Here's the drawing with two shaded views (mm, measured from the low corner). I have some questions. A direction names the side the tool comes from. Coordinates: 2 decimals unless noted, no trailing zeros. Write each loop counter-clockwise with the first axis right and the second up, starting at its lowest first coordinate (ties: lowest second). Pieces come first, ordered by that corner, then holes. Notation, with made-up numbers: (-14.75, 9) -> (-2.75, 9) arc R26 cw to (-2.75, 27) -> close; hole circle Ø5 at (22.5, 80). An arc over 180 degrees is marked (long way). Put each result on its own line as item: value. Start each with the question number.
Item 1: I want a section at C-C, the plane z = 35.5. List the corners of the cut face in (x, y) for me, then the cut area to 3 significant figures.
Item 2: If we mould it in two halves opening along Y, with no side actions, what happens to the marked faces 3, 4 and 5? For each: released by +Y, released by -Y, zero draft, split by the parting line, or undercut.
Item 3: I need wall thicknesses on line 1 (Z direction, x = 14.25, y = 75); line 2 (Z direction, x = 4.5, y = 100); line 3 (Y direction, x = 17.75, z = 50). Which ranges of each line are inside material? Lowest first, please. Write a range as [from, to].
Item 4: On a 3-axis mill with a long thin cutter (end or side, diameter ignored), from which of +Z, -Z, +X, -X, +Y, -Y can I reach the whole of each face in a straight line? I mean the marked faces 1 and 2. Say none if no direction works.
Item 5: I want a section at B-B, the plane x = 11.5. State how many separate pieces and enclosed holes the cut face has, then the cut area to 3 significant figures.
Item 6: I want a section at A-A, the plane x = 17.75. List the corners of the cut face in (y, z) for me.
Item 7: For pin 1 (9.5 mm diameter, centred on y = 50, z = 75, fed in from +X); pin 2 (11 mm diameter, centred on y = 100, z = 100, fed in from -X); pin 3 (4 mm diameter, centred on x = 17.5, z = 60, fed in from +Y), each with a flat end and sliding along its axis, tell me the tip position at first contact or that it passes through.
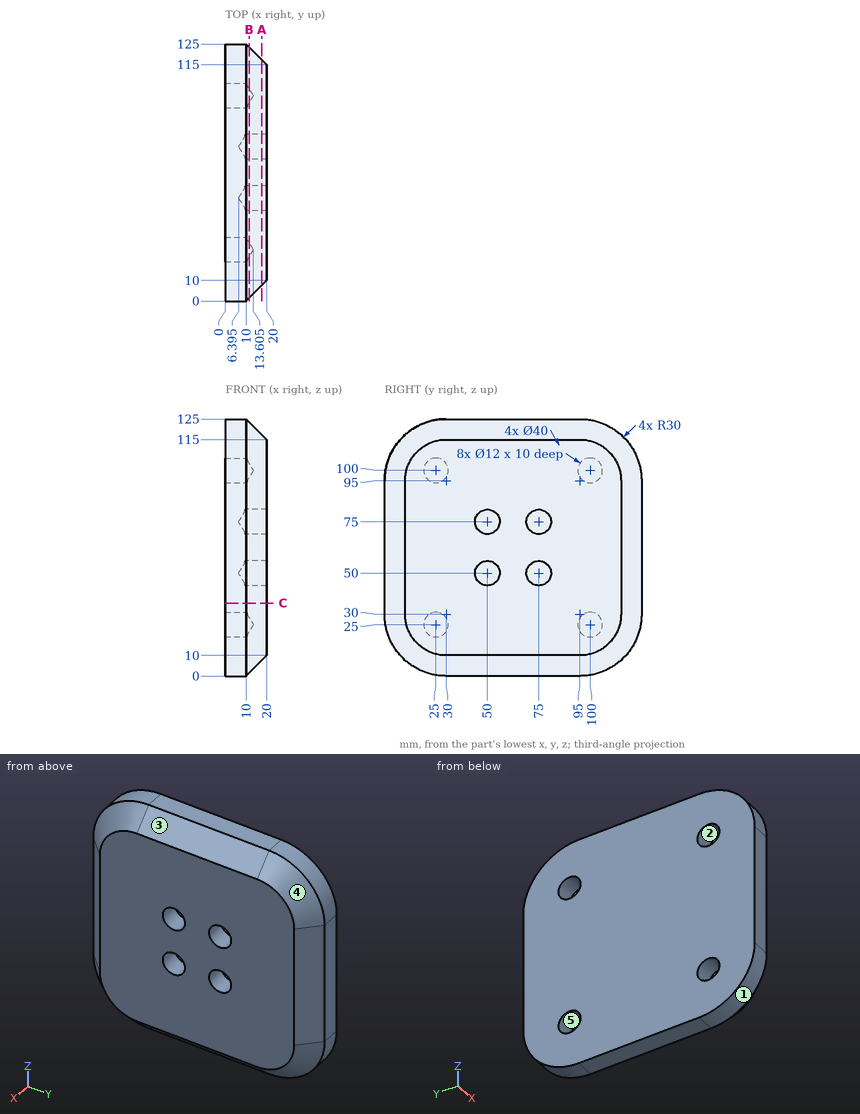
Calculated:
1. outline: (0, 0) -> (10, 0) -> (20, 10) -> (20, 115) -> (10, 125) -> (0, 125) -> close
1. area: 2,400 mm2
2. face 3: zero draft
2. face 4: released by +Y
2. face 5: undercut
3. line 1: z = [4.25, 44], [56, 69], [81, 120.75]
3. line 2: z = [0.42, 19], [31, 94], [106, 124.58]
3. line 3: y = [7.75, 44], [56, 69], [81, 117.25]
4. face 1: -Z, +X, -X, -Y
4. face 2: -X
5. separate pieces: 1
5. enclosed holes: 8
5. area: 13,600 mm2
6. outline: (7.75, 30) arc R22.25 ccw to (30, 7.75) -> (95, 7.75) arc R22.25 ccw to (117.25, 30) -> (117.25, 95) arc R22.25 ccw to (95, 117.25) -> (30, 117.25) arc R22.25 ccw to (7.75, 95) -> close; hole circle Ø12 at (50, 50); hole circle Ø12 at (50, 75); hole circle Ø12 at (75, 50); hole circle Ø12 at (75, 75)
7. pin 1: stops at x = 9.25
7. pin 2: stops at x = 10.3
7. pin 3: stops at y = 119.5
